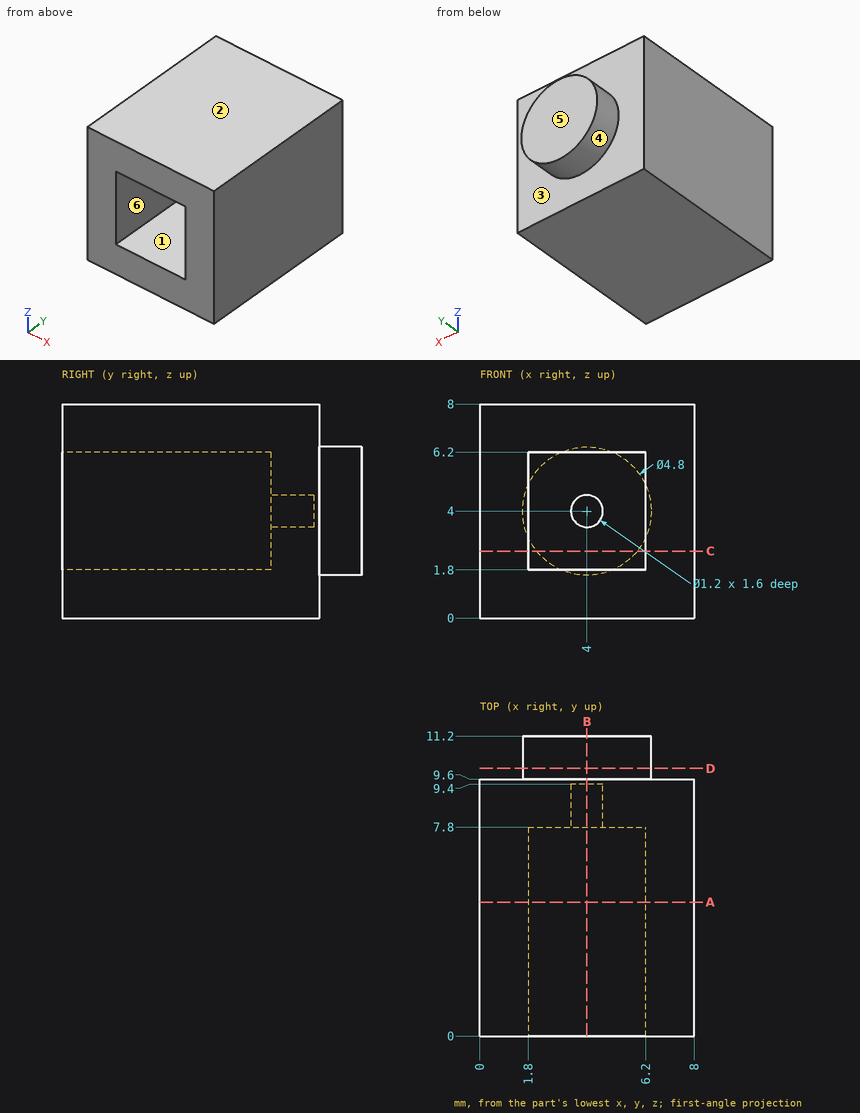
Design review of the part shown in the three views and the two pictorial views. Dimensions are in mm from the part's minimum x, y and z. A direction names the side the tool comes from. Coordinates: 2 decimals unless noted, no trailing zeros. Write each loop counter-clockwise with the first axis right and the second up, starting at its lowest first coordinate (ties: lowest second). Pieces come first, ordered by that corner, then holes.
(1) Tool access review of the marked faces 1, 2 and 3: name each direction out of +Z, -Z, +X, -X, +Y, -Y from which nothing blocks a thin tool from reaching the whole face with its end or side.
(2) Wall thickness on probe 1 along Z at (x, y) = (4, 9); probe 2 along X at (y, z) = (7.75, 4.25): over which ranges is each line inside the solid? List them lowest first.
(3) For pin 1 Ø1.3 at (x, z) = (3.5, 3.5) entering from -Y, flat-tipped, find the tip position at first contact; note if it passes through.
(4) The part is to be moulded in two halves that separate along Z. For the marked faces 4, 5 and 6, say which applies: +Z half, -Z half, draft (parallel to the pull), parting line (faces both ways), or undercut.
(5) Add section C-C on z = 2.5. Give the boundary of the cut face in (x, y).
(6) Add section A-A on y = 5. Give the boundary of the cut face in (x, z).
(7) Add section B-B on x = 4. Give the boundary of the cut face in (y, z).
(8) Add section D-D on y = 10. Give the boundary of the cut face in (x, z).
Answer sheet:
1. face 1: -Y
1. face 2: +Z, +X, -X, +Y, -Y
1. face 3: +Y
2. probe 1: z = 0 to 3.4, 4.6 to 8
2. probe 2: x = 0 to 1.8, 6.2 to 8
3. pin 1: stops at y = 7.8
4. face 4: parting line
4. face 5: draft
4. face 6: undercut
5. outline: (0, 0) - (1.8, 0) - (1.8, 7.8) - (6.2, 7.8) - (6.2, 0) - (8, 0) - (8, 9.6) - (5.87, 9.6) - (5.87, 11.2) - (2.13, 11.2) - (2.13, 9.6) - (0, 9.6) - close
6. outline: (0, 0) - (8, 0) - (8, 8) - (0, 8) - close; hole (1.8, 1.8) - (6.2, 1.8) - (6.2, 6.2) - (1.8, 6.2) - close
7. outline: (0, 0) - (9.6, 0) - (9.6, 1.6) - (11.2, 1.6) - (11.2, 6.4) - (9.6, 6.4) - (9.6, 8) - (0, 8) - (0, 6.2) - (7.8, 6.2) - (7.8, 4.6) - (9.4, 4.6) - (9.4, 3.4) - (7.8, 3.4) - (7.8, 1.8) - (0, 1.8) - close
8. outline: circle Ø4.8 at (4, 4)
